Solid Edge part; units mm, degrees
sketch "Sketch1" plane through (0, 0, 0) normal (0, 0, 1) x (1, 0, 0)
  line L0 (-2.7579, 81.4753) -> (-7.1387, 75.7615)
  line L1 (-7.1387, 75.7615) -> (-4.3808, 69.1106)
  line L2 (-4.3808, 69.1106) -> (2.7579, 68.1737)
  line L3 (2.7579, 68.1737) -> (7.1387, 73.8875)
  line L4 (7.1387, 73.8875) -> (4.3808, 80.5384)
  line L5 (4.3808, 80.5384) -> (-2.7579, 81.4753)
extrude "Protrusion1" add sketch "Sketch1" along normal up to vertex (5.6 mm away)
sketch "Sketch2" plane through (0, 74.8245, 5.6) normal (0, 0, 1) x (0.383, -0.9237, 0)
  circle A0 centre (0, 0) radius 4.2
extrude "Protrusion2" add sketch "Sketch2" along normal blind 70
sketch "Sketch3" plane through (0, 74.8245, 0) normal (0, -1, 0) x (1, 0, 0)
  circle A0 centre (-4.2, 45.1) radius 1.5
revolve "RevolvedCutout1" cut sketch "Sketch3" angle 360 about axis through (0, 74.8245, 54) along (0, 0, -1)
Check sheet for the modelled part. Datum: model origin and axes. Units: mm. A direction names the side the tool comes from. Round coordinates to 2 decimals unless told otherwise and drop trailing zeros. Loops run counter-clockwise (first coordinate to the right, second up) from the corner with the lowest first, then second, coordinate; pieces in that order, holes last. Notation, with made-up numbers: (44, 11) - (49, 11) arc R21 ccw to (49, 38) - close; hole circle Ø11 at (38.25, 28.25). An arc over 180 degrees is marked (long way). Answer as a JSON object with one key per item and string values. Group by question number.
Q1. Sectioned sample at A-A, the plane x = 0. Enter the section's corners in (y, z).
Q2. Scan lines: line 1 along Z through (x, y) = (5.25, 77.75); line 2 along Y through (x, z) = (0.25, 69.5); line 3 along Z through (x, y) = (0, 71). Record each from-to range of solid material in increasing order. Write a range as [from, to].
Q3. Mould release check, pull along Z, two halves, no side actions. Record for faces 1 (the face through (0, 75, 0)), 2 (the face through (0.86, 81, 2.76)), 3 (the face through (0, 70, 5.6)): released by +Z, released by -Z, zero draft, split by the parting line, or undercut.
Q4. Set-up check for faces 4 (the face through (-0.86, 68.65, 2.76)), 5 (the face through (-2.407, 71.382, 24.334)): record each of +Z, -Z, +X, -X, +Y, -Y from which the full face is reachable in a straight line by a thin tool's end or side.
Q5. Gauge pin test, flat ends, axial feed: P1, Ø8, axis at x = -0.5, z = 25.5, coming from the +Y side; P2, Ø1.5, axis at y = 74, z = 11.5, coming from the -X side; P3, Ø1, axis at x = -2, z = 54, coming from the +Y side. Record the tip position at first contact, or that the pin passes through.
Solution:
{
 "1": {"outline": "(68.54, 0) - (81.11, 0) - (81.11, 5.6) - (79.02, 5.6) - (79.02, 43.6) arc R1.5 cw to (79.02, 46.6) - (79.02, 75.6) - (70.62, 75.6) - (70.62, 46.6) arc R1.5 cw to (70.62, 43.6) - (70.62, 5.6) - (68.54, 5.6) - close"},
 "2": {"line 1": "z = [0, 5.6]", "line 2": "y = [70.63, 79.02]", "line 3": "z = [0, 43.65], [46.55, 75.6]"},
 "3": {"face 1": "released by -Z", "face 2": "zero draft", "face 3": "released by +Z"},
 "4": {"face 4": "+Z, -Z, -X, -Y", "face 5": "+Z"},
 "5": {"P1": "stops at y = 79.02", "P2": "stops at x = -4.2", "P3": "stops at y = 78.75"}
}
